Could you check a few things on this drawing? It's one solid part, dimensions in mm from its lowest x, y, z. A direction names the side the tool comes from. Give positions to 0.01 mm unless a question says otherwise; leave off trailing zeros. Loops run counter-clockwise (first coordinate to the right, second up) from the corner with the lowest first, then second, coordinate; pieces in that order, holes last.
Q1. I'm going to push flat-ended pins straight in: P1, Ø1, axis at y = 8.5, z = 20.5, coming from the +X side; P2, Ø2, axis at x = 5.5, z = 17, coming from the -Y side; P3, Ø4, axis at x = 3, z = 6.5, coming from the +Y side. Where does each tip first touch, or does it pass through?
Q2. Suppose I cut it at C-C (z = 26). List the corners of the cut face in (x, y) for me, and give its area (3 significant figures).
Q3. Suppose I cut it at A-A (x = 5). List the corners of the cut face in (y, z) for me, and give its area (3 significant figures).
Q4. Suppose I cut it at D-D (x = 9.25). List the corners of the cut face in (y, z) for me, and give its area (3 significant figures).
Q5. For the marked faces 1, 2 and 3, which set-ups out of +Z, -Z, +X, -X, +Y, -Y let a thin tool reach every point of the face, with its end or its side?
Q6. I need wall thicknesses on probe 1 along Z at (x, y) = (0.5, 6); probe 2 along Z at (x, y) = (2, 7); probe 3 along X at (y, z) = (3.75, 23). Which ranges of each line are inside material? Lowest first, please.
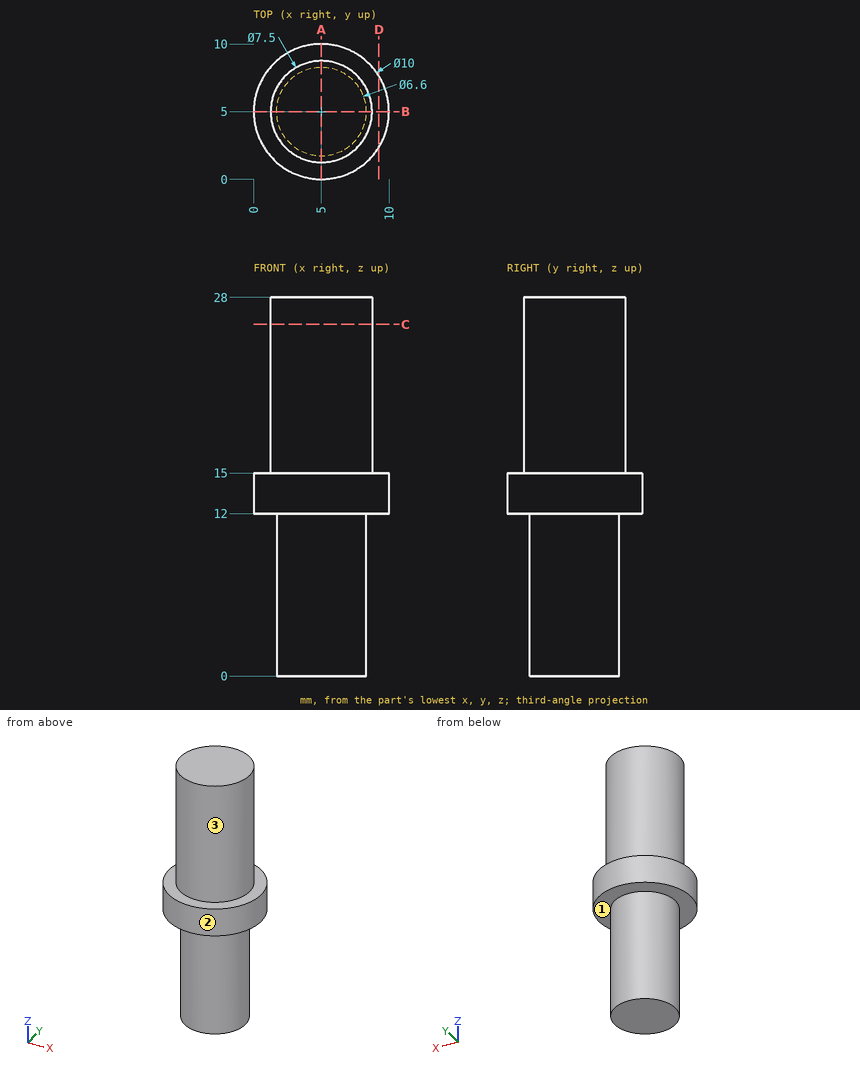
Solutions:
1. P1: stops at x = 7.25
1. P2: stops at y = 1.25
1. P3: stops at y = 8.3
2. outline: circle Ø7.5 at (5, 5)
2. area: 44.2 mm2
3. outline: (0, 12) - (1.7, 12) - (1.7, 0) - (8.3, 0) - (8.3, 12) - (10, 12) - (10, 15) - (8.75, 15) - (8.75, 28) - (1.25, 28) - (1.25, 15) - (0, 15) - close
3. area: 207 mm2
4. outline: (2.37, 12) - (7.63, 12) - (7.63, 15) - (2.37, 15) - close
4. area: 15.8 mm2
5. face 1: -Z
5. face 2: +Z, -Z
5. face 3: +Z
6. probe 1: z = 12 to 15
6. probe 2: z = 12 to 28
6. probe 3: x = 1.46 to 8.54
